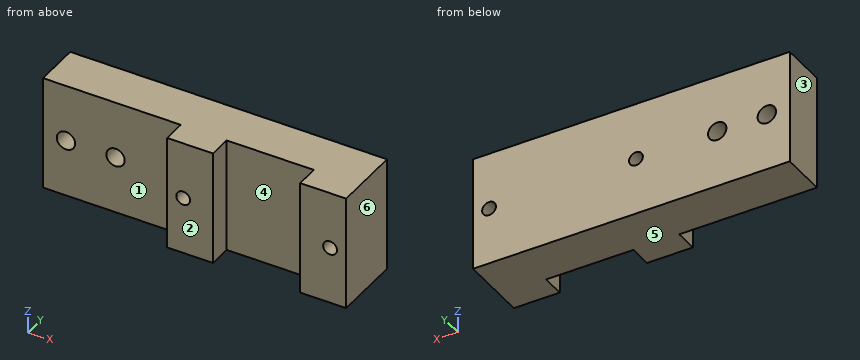
Autodesk Inventor part; units mm, degrees
ref_plane "YZ Plane" through (0, 0, 0) normal (1, 0, 0) x (0, 1, 0)
ref_plane "XZ Plane" through (0, 0, 0) normal (0, 1, 0) x (-1, 0, 0)
ref_plane "XY Plane" through (0, 0, 0) normal (0, 0, 1) x (1, 0, 0)
sketch "Sketch1" plane through (0, 0, 0) normal (0, 0, 1) x (1, 0, 0)
  line L0 (-10, 10) -> (-10, 20)
  line L1 (-10, 20) -> (59, 20)
  line L2 (59, 20) -> (59, 5)
  line L3 (59, 5) -> (49, 5)
  line L4 (49, 5) -> (49, 10)
  line L5 (49, 10) -> (30, 10)
  line L6 (30, 10) -> (30, 5)
  line L7 (30, 5) -> (20, 5)
  line L8 (20, 5) -> (20, 10)
  line L9 (20, 10) -> (-10, 10)
  point P0 (0, 0)
  dimension "d0" = 19
  dimension "d1" = 10
  dimension "d2" = 10
  dimension "d3" = 30
  dimension "d4" = 10
  dimension "d5" = 5
  dimension "d6" = 59
  dimension "d7" = 10
extrude "Extrusion1" add sketch "Sketch1" along normal mid plane 25
sketch "Sketch2" plane through (-10, 20, 12.5) normal (0, 1, 0) x (1, 0, 0)
  circle A0 centre (5, 12.5) radius 2
  circle A1 centre (15.8, 12.5) radius 2
  line L0 (30, 25) -> (30, 0)
  line L1 (0, 25) -> (69, 25)
  line L2 (0, 0) -> (0, 25)
  circle A2 centre (65.5, 12.5) radius 1.5
  line L3 (69, 25) -> (69, 0)
  circle A3 centre (33.5, 12.5) radius 1.5
  point P0 (10, 12.5)
  dimension "d10" = 4
  dimension "d11" = 4
  dimension "d15" = 12.5
  dimension "d16" = 12.5
  dimension "d19" = 5
  dimension "d20" = 10.8
  dimension "d22" = 3
  dimension "d24" = 3.5
  dimension "d26" = 12.5
  dimension "d28" = 12.5
  dimension "d29" = 3
  dimension "d30" = 3.5
extrude "Extrusion2" cut sketch "Sketch2" against normal blind 15
properties part number "Load Cell holder" material "ABS Plastic"
The model under review builds one solid part; all positions refer to its coordinate system, in mm. Face numbers are marked on the shaded views. A direction names the side the tool comes from. Give positions to 0.01 mm unless a question says otherwise; leave off trailing zeros. Loops run counter-clockwise (first coordinate to the right, second up) from the corner with the lowest first, then second, coordinate; pieces in that order, holes last. Notation, with made-up numbers: (28.25, -18) - (53.25, -18) arc R17 ccw to (53.25, -7) - close; hole circle Ø3 at (76.25, 6). An arc over 180 degrees is marked (long way). Answer as a JSON object with one key per item and string values.
Q1. Insertion check: pin 1 (5.5 mm diameter, centred on y = 6.5, z = 5.5, fed in from -X); pin 2 (1 mm diameter, centred on x = 17, z = -1, fed in from -Y); pin 3 (3 mm diameter, centred on x = -5, z = 0, fed in from -Y). Each pin has a flat end and moves straight along its axis. Give the tip position at first contact, or say it passes through.
Worked out:
{"pin 1": "stops at x = 20", "pin 2": "stops at y = 10", "pin 3": "passes through"}
Q2. Add section B-B on z = 0. State the section outline as (x, y) points, plus the area to 3 significant figures.
Worked out:
{"outline": "(-10, 10) - (-7, 10) - (-7, 20) - (-10, 20) - close; (-3, 10) - (3.8, 10) - (3.8, 20) - (-3, 20) - close; (7.8, 10) - (20, 10) - (20, 5) - (22, 5) - (22, 20) - (7.8, 20) - close; (25, 5) - (30, 5) - (30, 10) - (49, 10) - (49, 5) - (54, 5) - (54, 20) - (25, 20) - close; (57, 5) - (59, 5) - (59, 20) - (57, 20) - close", "area": "620 mm^2"}
Q3. Add section A-A on x = 55.5. State the section outline as (y, z) points.
Worked out:
{"outline": "(5, -12.5) - (20, -12.5) - (20, -1.5) - (5, -1.5) - close; (5, 1.5) - (20, 1.5) - (20, 12.5) - (5, 12.5) - close"}
Q4. Add section D-D on y = 14.75. State the section outline as (x, z) points.
Worked out:
{"outline": "(-10, -12.5) - (59, -12.5) - (59, 12.5) - (-10, 12.5) - close; hole circle Ø4 at (-5, 0); hole circle Ø4 at (5.8, 0); hole circle Ø3 at (23.5, 0); hole circle Ø3 at (55.5, 0)"}
Q5. To check wall thickness, follow line 1 along X through (y, z) = (9, 0); line 2 along X through (y, z) = (14, 0); line 3 along Z through (x, y) = (5.8, 15.5). State the ranges of each line that lie inside material, in increasing order.
Worked out:
{"line 1": "x = 20 to 22, 25 to 30, 49 to 54, 57 to 59", "line 2": "x = -10 to -7, -3 to 3.8, 7.8 to 22, 25 to 54, 57 to 59", "line 3": "z = -12.5 to -2, 2 to 12.5"}
Q6. For the marked faces 1 and 2, list the 3-axis set-ups (+Z, -Z, +X, -X, +Y, -Y) from which the entire face can be reached by the end or side of a thin tool; tool diameter is ignored.
Worked out:
{"face 1": "+Z, -Z, -X, -Y", "face 2": "+Z, -Z, +X, -X, -Y"}
Q7. Add section C-C on y = 8. State the section outline as (x, z) points, plus the area to 3 significant figures.
Worked out:
{"outline": "(20, -12.5) - (30, -12.5) - (30, 12.5) - (20, 12.5) - close; (49, -12.5) - (59, -12.5) - (59, 12.5) - (49, 12.5) - close; hole circle Ø3 at (23.5, 0); hole circle Ø3 at (55.5, 0)", "area": "486 mm^2"}
Q8. Mouldability with a two-part tool opening along X and no side actions: class the marked faces 3, 4, 5 and 6 as +X half, -X half, draft (parallel to the pull), parting line (faces both ways), or undercut.
Worked out:
{"face 3": "-X half", "face 4": "undercut", "face 5": "draft", "face 6": "+X half"}
